Input: part model. Units: mm. Frame: model coordinates. Face numbers are marked on the shaded views. Round coordinates to 2 decimals unless told otherwise and drop trailing zeros. Loops run counter-clockwise (first coordinate to the right, second up) from the corner with the lowest first, then second, coordinate; pieces in that order, holes last. Notation, with made-up numbers: (80.5, -38.5) -> (101.5, -38.5) arc R37 cw to (101.5, -2.5) -> close; hole circle Ø1 at (81, -32). An arc over 180 degrees is marked (long way). Answer as a JSON object with one key per item and string values. Group by question number.
Item 1: Pin query (flat end, axial travel): pin 1 (1.5 mm diameter, centred on x = 13.5, z = -2.5, fed in from -Y); pin 2 (1.5 mm diameter, centred on y = -98, z = -13.5, fed in from +X); pin 3 (8 mm diameter, centred on y = -89.5, z = 23, fed in from -X). Return the tip coordinate at first contact, or that it passes through.
Item 2: Section query B-B on z = 0. Return loops of the section in (x, y), and give its area (3 significant figures).
Item 3: Draft query along Z for the marked faces 1, 2 and 3. Return one class per face: released by +Z, released by -Z, zero draft, split by the parting line, or undercut.
Item 4: Material intervals for line 1 (X direction, y = -76, z = 0); line 2 (Y direction, x = -15, z = 2), sorted ascending. Write a range as [from, to].
Item 5: Section query A-A on x = 0. Return loops of the section in (y, z), and give its area (3 significant figures).
Item 6: Section query D-D on x = -46.5. Return loops of the section in (y, z), and give its area (3 significant figures).
Item 7: Section query C-C on y = -40. Return loops of the section in (x, z), and give its area (3 significant figures).
from build123d import *

# Parameters (mm, degrees)
F0_R     = 40
F0_R_2   = 35
F1_DEPTH = 120
F2_R     = 55
F2_R_2   = 40
F2_R_3   = 35
F3_DEPTH = 5


with BuildPart() as f1:
    # F0 (on Front) → F1 (new body)
    with BuildSketch(Plane.XZ):
        Circle(F0_R)
        Circle(F0_R_2, mode=Mode.SUBTRACT)
    extrude(amount=F1_DEPTH)

    # F2 (on face) → F3 (join)
    with BuildSketch(Plane(origin=(0, 0, 0), x_dir=(-1, 0, 0), z_dir=(0, 1, 0))):
        Circle(F2_R)
        Circle(F2_R_2, mode=Mode.SUBTRACT)
        Circle(F2_R_2)
        Circle(F2_R_3, mode=Mode.SUBTRACT)
        Circle(F2_R_3)
    extrude(amount=-F3_DEPTH)


solid = f1.part
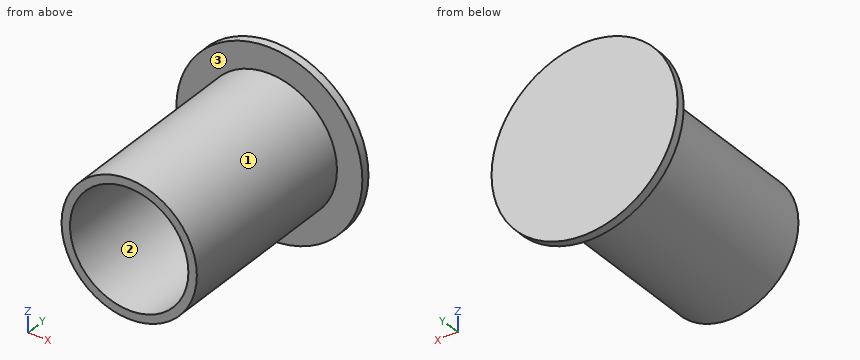
Solved:
{
 "1": {"pin 1": "y = -5", "pin 2": "x = 37.91", "pin 3": "x = -35.2"},
 "2": {"outline": "(-55, -5) -> (-40, -5) -> (-40, -120) -> (-35, -120) -> (-35, -5) -> (35, -5) -> (35, -120) -> (40, -120) -> (40, -5) -> (55, -5) -> (55, 0) -> (-55, 0) -> close", "area": "1,700 mm²"},
 "3": {"face 1": "split by the parting line", "face 2": "undercut", "face 3": "zero draft"},
 "4": {"line 1": "[-40, -35], [35, 40]", "line 2": "[-5, 0]"},
 "5": {"outline": "(-120, -40) -> (-5, -40) -> (-5, -55) -> (0, -55) -> (0, 55) -> (-5, 55) -> (-5, 40) -> (-120, 40) -> (-120, 35) -> (-5, 35) -> (-5, -35) -> (-120, -35) -> close", "area": "1,700 mm²"},
 "6": {"outline": "(-5, -29.37) -> (0, -29.37) -> (0, 29.37) -> (-5, 29.37) -> close", "area": "294 mm²"},
 "7": {"outline": "circle Ø80 at (0, 0); hole circle Ø70 at (0, 0)", "area": "1,180 mm²"}
}
